Geometry check sheet. Reference: the model listing, model coordinates, mm. A direction names the side the tool comes from. Round coordinates to 2 decimals unless told otherwise and drop trailing zeros. Order: outer loops, then holes, each group sorted by start corner. A loop starts at its lowest first (then second) coordinate and runs counter-clockwise, first axis right, second up. Notation, with made-up numbers: (41, 23.25) - (71, 23.25) arc R17 ccw to (71, 36.25) - close; hole circle Ø7 at (-32.75, 46.5). An arc over 180 degrees is marked (long way). One line per question, with ' | ' between items. Start each with the question number.
Q1. Tool access check on faces 1 (the face through (6.25, -10.77, 4.55)), 2 (the face through (9.2, 6.3, 0)). Record the directions out of +Z, -Z, +X, -X, +Y, -Y that give a thin tool (end or side, any length) a straight path to the whole face; none if there is none.
Q2. Sectioned sample at A-A, the plane z = -4.5. Enter the section's corners in (x, y).
Q3. Mould release check, pull along X, two halves, no side actions. Record for faces 3 (the face through (10.44, -5.92, 1.91)), 4 (the face through (0, -12, 2)), 5 (the face through (1.73, -7.81, -3.62)), 6 (the face through (-10.44, 5.92, 1.91)): +X half, -X half, draft (parallel to the pull), parting line (faces both ways), or undercut.
Q4. Gauge pin test, flat ends, axial feed: P1, Ø13, axis at x = 0, y = 0, coming from the -Z side; P2, Ø2, axis at y = 5, z = -0.5, coming from the +X side; P3, Ø1.5, axis at y = 6.5, z = 0.5, coming from the +X side; P4, Ø3, axis at y = -4.5, z = -0.5, coming from the -X side. Record the tip position at first contact, or that the pin passes through.
Q5. Material ranges on line 1 along Y through (x, z) = (0, -6.75); line 2 along Z through (x, y) = (11.5, 1.75); line 3 along Y through (x, z) = (3, -3.5), recorded low to high.
Autodesk Inventor part; units mm, degrees
ref_plane "YZ Plane" through (0, 0, 0) normal (1, 0, 0) x (0, 1, 0)
ref_plane "XZ Plane" through (0, 0, 0) normal (0, 1, 0) x (-1, 0, 0)
ref_plane "XY Plane" through (0, 0, 0) normal (0, 0, 1) x (1, 0, 0)
sketch "Sketch1" plane through (0, 0, 0) normal (0, 0, 1) x (1, 0, 0)
  line L0 (-6.9282, -12) -> (-13.8564, 0)
  line L1 (-13.8564, 0) -> (-6.9282, 12)
  line L2 (-6.9282, 12) -> (6.9282, 12)
  line L3 (6.9282, 12) -> (13.8564, 0)
  line L4 (13.8564, 0) -> (6.9282, -12)
  line L5 (6.9282, -12) -> (-6.9282, -12)
  circle A0 centre (0, 0) radius 12
  circle A1 centre (0, 0) radius 7
  dimension "d0" = 24
  dimension "d1" = 24
  dimension "d2" = 14
extrude "Extrusion1" add sketch "Sketch1" along normal blind 5 contours L0 A0 L5 | L0 L1 A0 | A0 | A0 L4 L5 | L1 L2 A0 | A0 L3 L4 | L2 L3 A0 | A1
sketch "Sketch2" plane through (0, 0, 5) normal (0, 0, 1) x (1, 0, 0)
  circle A0 centre (0, 0) radius 12
  dimension "d5" = 24
extrude "Extrusion2" cut sketch "Sketch2" against normal blind 5 draft 45 keep common part
sketch "Sketch3" plane through (0, 0, 0) normal (0, 0, -1) x (-1, 0, 0)
  circle A0 centre (0, 0) radius 11
  circle A1 centre (0, 0) radius 8
  dimension "d8" = 22
  dimension "d9" = 16
extrude "Extrusion3" add sketch "Sketch3" along normal blind 12
extrude "Extrusion4" cut sketch "Sketch3" against normal through all contours A1
thread "Thread1"
chamfer "Chamfer1" distance 1 angle 45 1 edges at (11, 0, -12)
equation "\"BendRadius\" = Thickness"
equation "\"BendReliefWidth\" = Thickness"
equation "\"BendReliefDepth\" = 0.5 * Thickness"
equation "\"CornerReliefSize\" = 4 * Thickness"
equation "\"MinimumRemnant\" = 2 * Thickness"
equation "\"TransitionRadius\" = BendRadius"
equation "\"JacobiRadiusSize\" = BendRadius"
equation "\"GapSize\" = Thickness"
properties part number "Hex.nut"
Determined:
1) face 1: +Z, +X, -Y | face 2: -Z
2) outline: circle Ø22 at (0, 0); hole circle Ø16 at (0, 0)
3) face 3: +X half | face 4: draft | face 5: undercut | face 6: -X half
4) P1: passes through | P2: stops at x = 11.47 | P3: stops at x = 10.54 | P4: stops at x = -12.07
5) line 1: y = -11 to -8, 8 to 11 | line 2: z = 0 to 5 | line 3: y = -10.58 to -7.42, 7.42 to 10.58
